```python
from build123d import *

# Parameters (mm, degrees)
F1_DEPTH  = 12.7
F2_R      = 6.35
F3_T      = -2.54
F4_R      = 3.175
F5_DEPTH  = 73.66
F7_R      = 3.175
F8_DEPTH  = 10.16
F9_R      = 1.5875
F10_DEPTH = 6.35


with BuildPart() as f1:
    # F0 (on Top) → F1 (new body)
    with BuildSketch(Plane.XY):
        with BuildLine():
            Line((-31.75, -31.75), (31.75, -31.75))
            ThreePointArc((31.75, -31.75), (36.2401280605, -29.8901280605), (38.1, -25.4))
            Line((38.1, -25.4), (38.1, 25.4))
            ThreePointArc((38.1, 25.4), (36.2401280605, 29.8901280605), (31.75, 31.75))
            Line((31.75, 31.75), (-31.75, 31.75))
            ThreePointArc((-31.75, 31.75), (-36.2401280605, 29.8901280605), (-38.1, 25.4))
            Line((-38.1, 25.4), (-38.1, -25.4))
            ThreePointArc((-38.1, -25.4), (-36.2401280605, -29.8901280605), (-31.75, -31.75))
        make_face()
    extrude(amount=F1_DEPTH)

    # F2
    f2_edges = [f1.edges().sort_by_distance(p)[0] for p in [
        (0, -31.75, 12.7),
        (36.240128, -29.890128, 12.7),
        (38.1, 0, 12.7),
        (36.240128, 29.890128, 12.7),
        (0, 31.75, 12.7),
        (-36.240128, 29.890128, 12.7),
        (-38.1, 0, 12.7),
        (-36.240128, -29.890128, 12.7),
    ]]
    fillet(f2_edges, radius=F2_R)

    # F3
    f3_openings = [f1.faces().sort_by_distance(p)[0] for p in [
        (0, 0, 0),
    ]]
    offset(amount=F3_T, openings=f3_openings)

    # F4 (on face) → F5 (cut, through all)
    with BuildSketch(Plane.YZ.offset(38.1)):
        with Locations((-19.05, 0)):
            Circle(F4_R)
    extrude(amount=-F5_DEPTH, mode=Mode.SUBTRACT)

    # F7 (on offset) → F8 (join, through all)
    with BuildSketch(Plane(origin=(0, 0, 10.16), x_dir=(1, 0, 0), z_dir=(0, 0, -1))):
        with Locations((-31.5977446735, 25.4)):
            Circle(F7_R)
        with Locations((-31.5977446735, -25.4)):
            Circle(F7_R)
        with Locations((31.9022553265, 25.4)):
            Circle(F7_R)
        with Locations((31.9022553265, -25.4)):
            Circle(F7_R)
    extrude(amount=F8_DEPTH)

    # F9 (on face) → F10 (cut)
    with BuildSketch(Plane(origin=(0, 0, 0), x_dir=(1, 0, 0), z_dir=(0, 0, -1))):
        with Locations((-31.5977446735, 25.4)):
            Circle(F9_R)
        with Locations((-31.5977446735, -25.4)):
            Circle(F9_R)
        with Locations((31.9022553265, 25.4)):
            Circle(F9_R)
        with Locations((31.9022553265, -25.4)):
            Circle(F9_R)
    extrude(amount=-F10_DEPTH, mode=Mode.SUBTRACT)


solid = f1.part
```
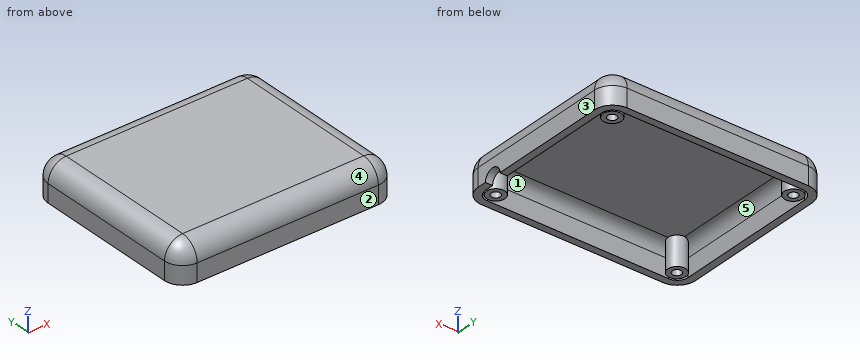
Geometry check sheet. Reference: the model listing, model coordinates, mm. Face numbers are marked on the shaded views. A direction names the side the tool comes from. Give positions to 0.01 mm unless a question says otherwise; leave off trailing zeros. Loops run counter-clockwise (first coordinate to the right, second up) from the corner with the lowest first, then second, coordinate; pieces in that order, holes last. Notation, with made-up numbers: M 46,33.25 L 91,33.25 A18 ccw 91,50.25 Z; hole C 30.5,-12.75 d8. An arc over 180 degrees is marked long. Write item = value, one per line.
(1) Tool access check on the marked faces 4 and 5. Record the directions out of +Z, -Z, +X, -X, +Y, -Y that give a thin tool (end or side, any length) a straight path to the whole face; none if there is none.
Answer below:
face_4 = +Z, +X, -X, -Y
face_5 = -Z
(2) Sectioned sample at B-B, the plane y = 18. Record the cut outline in (x, z), plus the area to 3 significant figures.
Answer below:
outline = M -38.1,0 L -35.56,0 L -35.56,6.35 A3.81 cw -31.75,10.16 L 31.75,10.16 A3.81 cw 35.56,6.35 L 35.56,0 L 38.1,0 L 38.1,6.35 A6.35 ccw 31.75,12.7 L -31.75,12.7 A6.35 ccw -38.1,6.35 Z
area = 234 mm2
(3) Sectioned sample at A-A, the plane x = 14.5. Record the cut outline in (y, z), plus the area to 3 significant figures.
Answer below:
outline = M -31.75,0 L -29.21,0 L -29.21,6.35 A3.81 cw -25.4,10.16 L 25.4,10.16 A3.81 cw 29.21,6.35 L 29.21,0 L 31.75,0 L 31.75,6.35 A6.35 ccw 25.4,12.7 L -25.4,12.7 A6.35 ccw -31.75,6.35 Z
area = 202 mm2
(4) Release check for a two-part mould opening along X. For the marked faces 1, 2 and 3 record: released by +X, released by -X, zero draft, split by the parting line, or undercut.
Answer below:
face_1 = undercut
face_2 = zero draft
face_3 = released by +X
(5) Gauge pin test, flat ends, axial feed: pin 1 Ø1.6 at (x, y) = (-32, -26) entering from -Z; pin 2 Ø6 at (x, y) = (8, 13) entering from -Z. Record the tip position at first contact, or that the pin passes through.
Answer below:
pin_1 = 6.35
pin_2 = 10.16
(6) Material ranges on line 1 (X direction, y = 25.4, z = 2); line 2 (X direction, y = 3.5, z = 5.75); line 3 (Y direction, x = -34.5, z = 8.5), recorded low to high. Write a range as [from, to].
Answer below:
line_1 = [-38.1, -35.56], [-34.77, -33.19], [-30.01, -28.42], [28.73, 30.31], [33.49, 35.08], [35.56, 38.1]
line_2 = [-38.1, -35.56], [35.56, 38.1]
line_3 = [-30.7, -26.93], [-26.69, -24.11], [24.11, 26.69], [26.93, 30.7]
